from build123d import *

# Parameters (mm, degrees)
SKETCH1_W           = 101.6
SKETCH1_H           = 50.8
BOSS_EXTRUDE1_DEPTH = 6.35
CUT_EXTRUDE2_REACH  = 59.15
SKETCH3_R           = 3.175
SKETCH3_R_2         = 2.667
FILLET1_R           = 6.35


with BuildPart() as part:
    # Sketch1 → Boss-Extrude1 (new body)
    with BuildSketch(Plane(origin=(0, 0, 0), x_dir=(1, 0, 0), z_dir=(0, 1, 0))):
        Rectangle(SKETCH1_W, SKETCH1_H)
    extrude(amount=BOSS_EXTRUDE1_DEPTH)

    # Sketch3 → Cut-Extrude2 (cut, up to next)
    with BuildSketch(Plane.XZ, mode=Mode.PRIVATE) as cut_extrude2_sk1:
        with Locations(Location((-38.1, 12.7, 0), (0, 0, 270))):
            Circle(SKETCH3_R)
    cut_extrude2_tool1 = extrude(cut_extrude2_sk1.sketch, amount=-CUT_EXTRUDE2_REACH, mode=Mode.PRIVATE) & part.part
    # Sketch3 → Cut-Extrude2 (cut, up to next)
    with BuildSketch(Plane.XZ, mode=Mode.PRIVATE) as cut_extrude2_sk2:
        with Locations(Location((-38.1, -12.7, 0), (0, 0, 90))):
            Circle(SKETCH3_R)
    cut_extrude2_tool2 = extrude(cut_extrude2_sk2.sketch, amount=-CUT_EXTRUDE2_REACH, mode=Mode.PRIVATE) & part.part
    # Sketch3 → Cut-Extrude2 (cut, up to next)
    with BuildSketch(Plane.XZ, mode=Mode.PRIVATE) as cut_extrude2_sk3:
        with Locations(Location((38.1, 12.7, 0), (0, 0, 90))):
            Circle(SKETCH3_R)
    cut_extrude2_tool3 = extrude(cut_extrude2_sk3.sketch, amount=-CUT_EXTRUDE2_REACH, mode=Mode.PRIVATE) & part.part
    # Sketch3 → Cut-Extrude2 (cut, up to next)
    with BuildSketch(Plane.XZ, mode=Mode.PRIVATE) as cut_extrude2_sk4:
        with Locations(Location((38.1, -12.7, 0), (0, 0, 270))):
            Circle(SKETCH3_R)
    cut_extrude2_tool4 = extrude(cut_extrude2_sk4.sketch, amount=-CUT_EXTRUDE2_REACH, mode=Mode.PRIVATE) & part.part
    # Sketch3 → Cut-Extrude2 (cut, up to next)
    with BuildSketch(Plane.XZ, mode=Mode.PRIVATE) as cut_extrude2_sk5:
        with Locations(Location((13.589, -12.75, 0), (0, 0, 90))):
            Circle(SKETCH3_R_2)
    cut_extrude2_tool5 = extrude(cut_extrude2_sk5.sketch, amount=-CUT_EXTRUDE2_REACH, mode=Mode.PRIVATE) & part.part
    # Sketch3 → Cut-Extrude2 (cut, up to next)
    with BuildSketch(Plane.XZ, mode=Mode.PRIVATE) as cut_extrude2_sk6:
        with Locations(Location((-13.589, -12.75, 0), (0, 0, 270))):
            Circle(SKETCH3_R_2)
    cut_extrude2_tool6 = extrude(cut_extrude2_sk6.sketch, amount=-CUT_EXTRUDE2_REACH, mode=Mode.PRIVATE) & part.part
    # Sketch3 → Cut-Extrude2 (cut, up to next)
    with BuildSketch(Plane.XZ, mode=Mode.PRIVATE) as cut_extrude2_sk7:
        with Locations(Location((13.589, 12.75, 0), (0, 0, 270))):
            Circle(SKETCH3_R_2)
    cut_extrude2_tool7 = extrude(cut_extrude2_sk7.sketch, amount=-CUT_EXTRUDE2_REACH, mode=Mode.PRIVATE) & part.part
    # Sketch3 → Cut-Extrude2 (cut, up to next)
    with BuildSketch(Plane.XZ, mode=Mode.PRIVATE) as cut_extrude2_sk8:
        with Locations(Location((-13.589, 12.75, 0), (0, 0, 90))):
            Circle(SKETCH3_R_2)
    cut_extrude2_tool8 = extrude(cut_extrude2_sk8.sketch, amount=-CUT_EXTRUDE2_REACH, mode=Mode.PRIVATE) & part.part
    add(cut_extrude2_tool1.solids().sort_by_distance((-38.1, 0, 12.7))[0], mode=Mode.SUBTRACT)
    add(cut_extrude2_tool2.solids().sort_by_distance((-38.1, 0, -12.7))[0], mode=Mode.SUBTRACT)
    add(cut_extrude2_tool3.solids().sort_by_distance((38.1, 0, 12.7))[0], mode=Mode.SUBTRACT)
    add(cut_extrude2_tool4.solids().sort_by_distance((38.1, 0, -12.7))[0], mode=Mode.SUBTRACT)
    add(cut_extrude2_tool5.solids().sort_by_distance((13.589, 0, -12.75))[0], mode=Mode.SUBTRACT)
    add(cut_extrude2_tool6.solids().sort_by_distance((-13.589, 0, -12.75))[0], mode=Mode.SUBTRACT)
    add(cut_extrude2_tool7.solids().sort_by_distance((13.589, 0, 12.75))[0], mode=Mode.SUBTRACT)
    add(cut_extrude2_tool8.solids().sort_by_distance((-13.589, 0, 12.75))[0], mode=Mode.SUBTRACT)

    # Fillet1
    fillet1_edges = [part.edges().sort_by_distance(p)[0] for p in [
        (50.8, 3.175, 25.4),
        (-50.8, 3.175, 25.4),
        (-50.8, 3.175, -25.4),
        (50.8, 3.175, -25.4),
    ]]
    fillet(fillet1_edges, radius=FILLET1_R)


solid = part.part
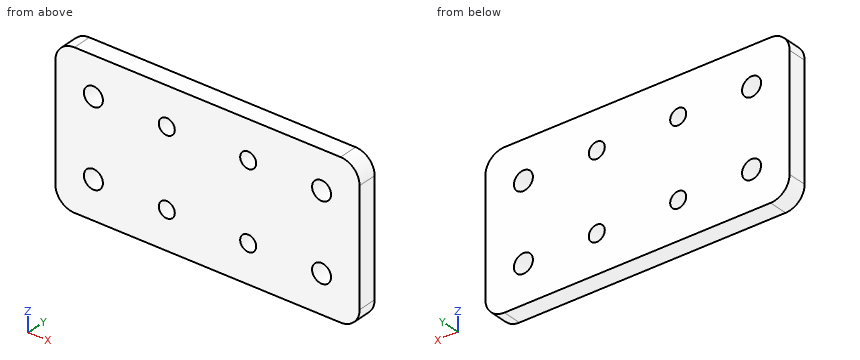
CAD build for the part. Positions are in the model's coordinates, mm. Give positions to 0.01 mm unless a question says otherwise; leave off trailing zeros. Loops run counter-clockwise (first coordinate to the right, second up) from the corner with the lowest first, then second, coordinate; pieces in that order, holes last. Notation, with made-up numbers: M 35.25,6 L 62.25,6 A6 cw 62.25,11 Z; hole C -2,-29 d1. An arc over 180 degrees is marked long. One line per question, with ' | ' between items. Start each with the question number.
1. Saw through at D-D on z = -12.75. Give the cut face in (x, y).
2. Saw through at B-B on z = 12.7. Give the cut face in (x, y) (3 decimals), plus the area to 3 significant figures.
3. Probe L1, parallel to X at y = 2.25, z = 12.75; L2, parallel to X at y = 4, z = 10.5; L3, parallel to Z at x = 38.5, y = 0.75. List the from-to ranges inside material, lowest first. Write a range as from..to.
4. Saw through at C-C on y = 3. State how many separate pieces and enclosed holes the cut face has, plus the area to 3 significant figures.
5. Flat gauge pins, fed straight in: pin 1 (5 mm diameter, centred on x = -13.589, z = -12.75, fed in from -Y); pin 2 (8.5 mm diameter, centred on x = -13.589, z = 12.75, fed in from +Y). Where does each tip first touch, or does it go through?
6. Saw through at A-A on x = -38.1. Give the cut face in (y, z) (3 decimals).
Result sheet:
1) outline: M -50.8,0 L -41.27,0 L -41.27,6.35 L -50.8,6.35 Z; M -34.93,0 L -16.26,0 L -16.26,6.35 L -34.93,6.35 Z; M -10.92,0 L 10.92,0 L 10.92,6.35 L -10.92,6.35 Z; M 16.26,0 L 34.93,0 L 34.93,6.35 L 16.26,6.35 Z; M 41.27,0 L 50.8,0 L 50.8,6.35 L 41.27,6.35 Z
2) outline: M -50.8,0 L -41.275,0 L -41.275,6.35 L -50.8,6.35 Z; M -34.925,0 L -16.256,0 L -16.256,6.35 L -34.925,6.35 Z; M -10.922,0 L 10.922,0 L 10.922,6.35 L -10.922,6.35 Z; M 16.256,0 L 34.925,0 L 34.925,6.35 L 16.256,6.35 Z; M 41.275,0 L 50.8,0 L 50.8,6.35 L 41.275,6.35 Z | area: 497 mm^2
3) L1: x = -50.8..-41.27, -34.93..-16.26, -10.92..10.92, 16.26..34.93, 41.27..50.8 | L2: x = -50.8..-40.39, -35.81..-15.02, -12.16..12.16, 15.02..35.81, 40.39..50.8 | L3: z = -25.4..-15.85, -9.55..9.55, 15.85..25.4
4) separate pieces: 1 | enclosed holes: 8 | area: 4,910 mm^2
5) pin 1: passes through | pin 2: stops at y = 6.35
6) outline: M 0,-25.4 L 6.35,-25.4 L 6.35,-15.875 L 0,-15.875 Z; M 0,-9.525 L 6.35,-9.525 L 6.35,9.525 L 0,9.525 Z; M 0,15.875 L 6.35,15.875 L 6.35,25.4 L 0,25.4 Z
